Read the model definition and answer for the solid it produces. Units are mm, in the model's axes. A direction names the side the tool comes from. Round coordinates to 2 decimals unless told otherwise and drop trailing zeros. Order: outer loops, then holes, each group sorted by start corner. A loop starts at its lowest first (then second) coordinate and runs counter-clockwise, first axis right, second up. Notation, with made-up numbers: (4.5, -6) -> (46.5, -6) arc R23 cw to (46.5, 14) -> close; hole circle Ø9 at (-4, 1). An arc over 180 degrees is marked (long way). Use a Markdown table: item, result. Add a question column.
1. For faces 1 (the face through (51.1, 21, -44)), 2 (the face through (47, 21, -52.9)), 3 (the face through (3, 21, -11)), 4 (the face through (27, -7, -22.4)), 5 (the face through (17, -7, -28)), determine the directions among +Z, -Z, +X, -X, +Y, -Y from which every point of the face is accessible in a straight line to the end or side of a thin tool.
2. Consider L1, parallel to Y at x = 38.5, z = -21.5; L2, parallel to Y at x = 45, z = -42.5; L3, parallel to Z at x = 33, y = -0.5. Determine where each line is inside the solid, lowest interval first. Write a range as [from, to].
3. Section A-A, the plane y = 20.5 is taken. Give the vertices of the cut face in (x, z).
4. Section D-D, the plane y = -2.5 is taken. Give the vertices of the cut face in (x, z).
5. Section B-B, the plane x = 7 is taken. Give the vertices of the cut face in (y, z).
6. Section C-C, the plane z = -12 is taken. Give the vertices of the cut face in (x, y), then the cut area to 3 significant figures.
7. Given pin 1 (12 mm diameter, centred on x = 28, y = -6.5, fed in from +Z); pin 2 (1 mm diameter, centred on y = -1, z = -32, fed in from -X); pin 3 (1.5 mm diameter, centred on x = 47.5, y = 21, fed in from +Z), each flat-ended and moving along its own axis, determine where each tip first touches the part or whether it passes through.
```python
from build123d import *

# Parameters (mm, degrees)
ESQUISSE1_W        = 54.1
ESQUISSE1_H        = 54.4
BOSS_EXTRU_1_DEPTH = 19
ESQUISSE2_W        = 20
ESQUISSE2_H        = 12
BOSS_EXTRU_2_DEPTH = 15
ESQUISSE3_W        = 9
ESQUISSE3_H        = 18
BOSS_EXTRU_3_DEPTH = 5


with BuildPart() as part:
    # Esquisse1 → Boss.-Extru.1 (new body)
    with BuildSketch(Plane(origin=(0, 0, 0), x_dir=(1, 0, 0), z_dir=(0, 1, 0))):
        with Locations((27.05, 27.2)):
            Rectangle(ESQUISSE1_W, ESQUISSE1_H)
    extrude(amount=BOSS_EXTRU_1_DEPTH)

    # Esquisse2 → Boss.-Extru.2 (add)
    with BuildSketch(Plane.XZ):
        with Locations((27, -28.4)):
            Rectangle(ESQUISSE2_W, ESQUISSE2_H)
    extrude(amount=BOSS_EXTRU_2_DEPTH)

    # Esquisse3 → Boss.-Extru.3 (add)
    with BuildSketch(Plane(origin=(0, 19, 0), x_dir=(1, 0, 0), z_dir=(0, 1, 0))):
        with Locations((46.6, 43.9)):
            Rectangle(ESQUISSE3_W, ESQUISSE3_H)
        with Locations((7.5, 11)):
            Rectangle(ESQUISSE3_W, ESQUISSE3_H)
    extrude(amount=BOSS_EXTRU_3_DEPTH)


solid = part.part
```
Verdict:
| question | item | result |
|---|---|---|
| 1 | face 1 | +Z, -Z, +X, +Y |
| 1 | face 2 | -Z, +X, -X, +Y |
| 1 | face 3 | +Z, -Z, -X, +Y |
| 1 | face 4 | +Z, +X, -X, -Y |
| 1 | face 5 | +Z, -Z, -X, -Y |
| 2 | L1 | y = [0, 19] |
| 2 | L2 | y = [0, 24] |
| 2 | L3 | z = [-34.4, -22.4] |
| 3 | outline | (3, -20) -> (12, -20) -> (12, -2) -> (3, -2) -> close; (42.1, -52.9) -> (51.1, -52.9) -> (51.1, -34.9) -> (42.1, -34.9) -> close |
| 4 | outline | (17, -34.4) -> (37, -34.4) -> (37, -22.4) -> (17, -22.4) -> close |
| 5 | outline | (0, -54.4) -> (19, -54.4) -> (19, -20) -> (24, -20) -> (24, -2) -> (19, -2) -> (19, 0) -> (0, 0) -> close |
| 6 | outline | (0, 0) -> (54.1, 0) -> (54.1, 19) -> (12, 19) -> (12, 24) -> (3, 24) -> (3, 19) -> (0, 19) -> close |
| 6 | area | 1,070 mm2 |
| 7 | pin 1 | stops at z = -22.4 |
| 7 | pin 2 | stops at x = 17 |
| 7 | pin 3 | stops at z = -34.9 |
